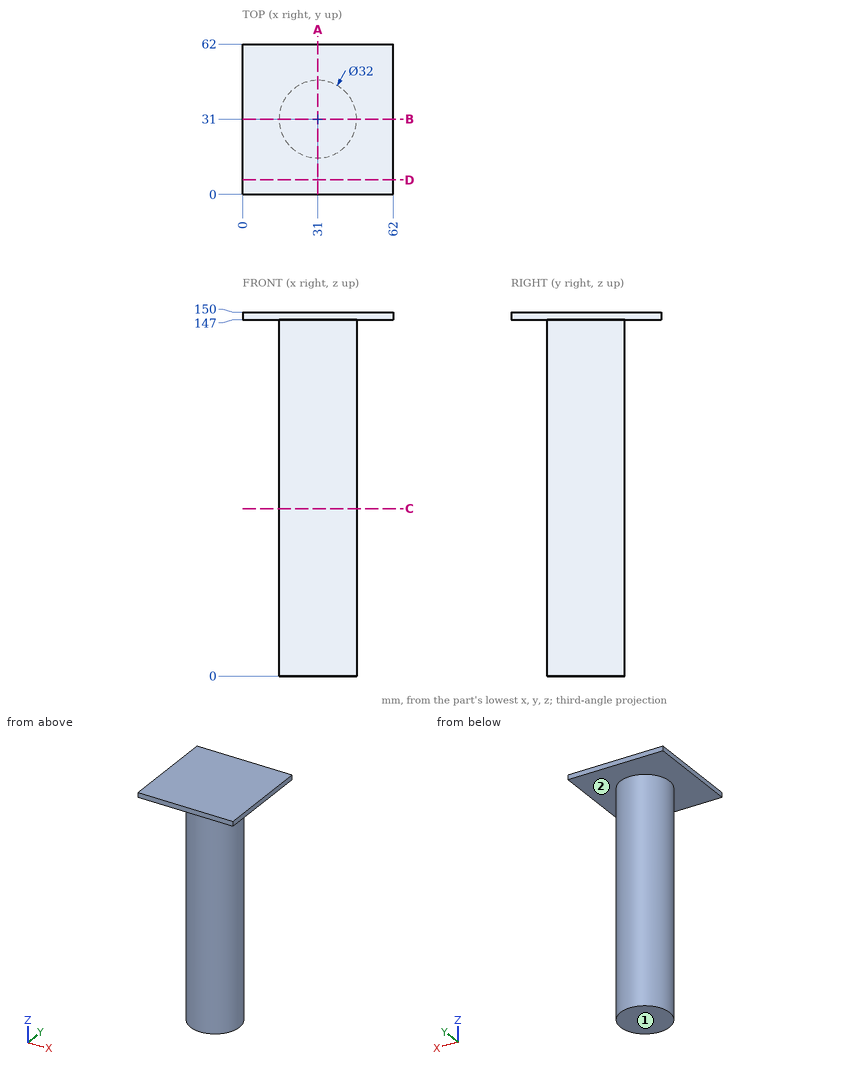
For this review, use the dimensioned drawing (mm, ordinates from the lowest corner) and the shaded views. A direction names the side the tool comes from. Coordinates: 2 decimals unless noted, no trailing zeros. Loops run counter-clockwise (first coordinate to the right, second up) from the corner with the lowest first, then second, coordinate; pieces in that order, holes last. Notation, with made-up numbers: (-35, 63.25) -> (11, 63.25) arc R13 ccw to (11, 84.25) -> close; hole circle Ø11 at (39, -29). An arc over 180 degrees is marked (long way). Use a Markdown table: item, result. Add a question column.
Item 1: Machinability: for the marked faces 1 and 2, which of the approach directions +Z, -Z, +X, -X, +Y, -Y give a long, thin tool a straight path to every point of the face, cutting with its end or side? Answer none if there is none.
Item 2: Wall thickness on L1, parallel to Z at x = 51.5, y = 52; L2, parallel to Y at x = 21, z = 129; L3, parallel to X at y = 23.5, z = 10.5: over which ranges is each line inside the solid? List them lowest first. Write a range as from..to.
Item 3: We need section A-A, the plane x = 31. Write out the cut boundary in (y, z), and give its area (3 significant figures).
Item 4: Clearance check with flat-ended pins moving along their axes: P1, Ø5, axis at y = 17, z = 79.5, coming from the -X side; P2, Ø12, axis at y = 47.5, z = 115, coming from the +X side; P3, Ø12, axis at x = 27, y = 8.5, coming from the -Z side. State where each tip first meets the part, or that it passes through.
Item 5: We need section D-D, the plane y = 6. Write out the cut boundary in (x, z), and give its area (3 significant figures).
Item 6: We need section C-C, the plane z = 69. Write out the cut boundary in (x, y), and give its area (3 significant figures).
Numbers:
| question | item | result |
|---|---|---|
| 1 | face 1 | -Z, +X, -X, +Y, -Y |
| 1 | face 2 | -Z |
| 2 | L1 | z = 147..150 |
| 2 | L2 | y = 18.51..43.49 |
| 2 | L3 | x = 16.87..45.13 |
| 3 | outline | (0, 147) -> (15, 147) -> (15, 0) -> (47, 0) -> (47, 147) -> (62, 147) -> (62, 150) -> (0, 150) -> close |
| 3 | area | 4,890 mm^2 |
| 4 | P1 | stops at x = 19.88 |
| 4 | P2 | stops at x = 43.07 |
| 4 | P3 | stops at z = 147 |
| 5 | outline | (0, 147) -> (62, 147) -> (62, 150) -> (0, 150) -> close |
| 5 | area | 186 mm^2 |
| 6 | outline | circle Ø32 at (31, 31) |
| 6 | area | 804 mm^2 |
